Here's how the part is built. I have some questions about the finished solid (model axes, mm). Face numbers are marked on the shaded views. Coordinates: 2 decimals unless noted, no trailing zeros. Loops run counter-clockwise (first coordinate to the right, second up) from the corner with the lowest first, then second, coordinate; pieces in that order, holes last.
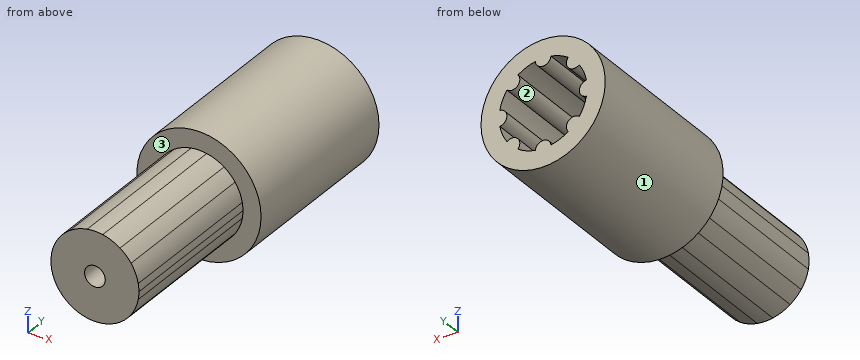
```python
from build123d import *

# Parameters (mm, degrees)
F0_R          = 6
F1_DEPTH      = 17
F0_R_2        = 2.5
F0_R_3        = 1
F2_DEPTH      = 15
F2_DEPTH_BACK = 3


with BuildPart() as f1:
    # F0 (on Front) → F1 (new body)
    with BuildSketch(Plane.XZ):
        Circle(F0_R)
        with BuildLine():
            ThreePointArc((4.183153, 0.75082), (4.233255, 0.376895), (4.25, 0))
            ThreePointArc((4.25, 0), (4.233255, -0.376895), (4.183153, -0.75082))
            ThreePointArc((4.183153, -0.75082), (3.926488, -1.626405), (3.488846, -2.427026))
            ThreePointArc((3.488846, -2.427026), (3.005204, -3.005204), (2.427026, -3.488846))
            ThreePointArc((2.427026, -3.488846), (1.626405, -3.926488), (0.75082, -4.183153))
            ThreePointArc((0.75082, -4.183153), (0, -4.25), (-0.75082, -4.183153))
            ThreePointArc((-0.75082, -4.183153), (-1.626405, -3.926488), (-2.427026, -3.488846))
            ThreePointArc((-2.427026, -3.488846), (-3.005204, -3.005204), (-3.488846, -2.427026))
            ThreePointArc((-3.488846, -2.427026), (-3.926488, -1.626405), (-4.183153, -0.75082))
            ThreePointArc((-4.183153, -0.75082), (-4.25, 0), (-4.183153, 0.75082))
            ThreePointArc((-4.183153, 0.75082), (-3.926488, 1.626405), (-3.488846, 2.427026))
            ThreePointArc((-3.488846, 2.427026), (-3.005204, 3.005204), (-2.427026, 3.488846))
            ThreePointArc((-2.427026, 3.488846), (-1.626405, 3.926488), (-0.75082, 4.183153))
            ThreePointArc((-0.75082, 4.183153), (0, 4.25), (0.75082, 4.183153))
            ThreePointArc((0.75082, 4.183153), (1.626405, 3.926488), (2.427026, 3.488846))
            ThreePointArc((2.427026, 3.488846), (3.005204, 3.005204), (3.488846, 2.427026))
            ThreePointArc((3.488846, 2.427026), (3.926488, 1.626405), (4.183153, 0.75082))
        make_face(mode=Mode.SUBTRACT)
        with BuildLine():
            ThreePointArc((4.183153, -0.75082), (4.233255, -0.376895), (4.25, 0))
            ThreePointArc((4.25, 0), (4.233255, 0.376895), (4.183153, 0.75082))
            ThreePointArc((4.183153, 0.75082), (3.496211, 0), (4.183153, -0.75082))
        make_face()
        with BuildLine():
            ThreePointArc((2.427026, 3.488846), (2.472194, 2.472194), (3.488846, 2.427026))
            ThreePointArc((3.488846, 2.427026), (3.005204, 3.005204), (2.427026, 3.488846))
        make_face()
        with BuildLine():
            ThreePointArc((-0.75082, 4.183153), (0, 3.496211), (0.75082, 4.183153))
            ThreePointArc((0.75082, 4.183153), (0, 4.25), (-0.75082, 4.183153))
        make_face()
        with BuildLine():
            ThreePointArc((-3.488846, 2.427026), (-2.472194, 2.472194), (-2.427026, 3.488846))
            ThreePointArc((-2.427026, 3.488846), (-3.005204, 3.005204), (-3.488846, 2.427026))
        make_face()
        with BuildLine():
            ThreePointArc((-4.183153, -0.75082), (-3.496211, 0), (-4.183153, 0.75082))
            ThreePointArc((-4.183153, 0.75082), (-4.25, 0), (-4.183153, -0.75082))
        make_face()
        with BuildLine():
            ThreePointArc((-3.488846, -2.427026), (-3.005204, -3.005204), (-2.427026, -3.488846))
            ThreePointArc((-2.427026, -3.488846), (-2.472194, -2.472194), (-3.488846, -2.427026))
        make_face()
        with BuildLine():
            ThreePointArc((-0.75082, -4.183153), (0, -4.25), (0.75082, -4.183153))
            ThreePointArc((0.75082, -4.183153), (0, -3.496211), (-0.75082, -4.183153))
        make_face()
        with BuildLine():
            ThreePointArc((2.427026, -3.488846), (3.005204, -3.005204), (3.488846, -2.427026))
            ThreePointArc((3.488846, -2.427026), (2.472194, -2.472194), (2.427026, -3.488846))
        make_face()
    extrude(amount=-F1_DEPTH)

    # F0 (on Front) → F2 (join, two sides)
    with BuildSketch(Plane.XZ) as f2_sk:
        with BuildLine():
            ThreePointArc((4.183153, -0.75082), (3.496211, 0), (4.183153, 0.75082))
            ThreePointArc((4.183153, 0.75082), (3.926488, 1.626405), (3.488846, 2.427026))
            ThreePointArc((3.488846, 2.427026), (2.472194, 2.472194), (2.427026, 3.488846))
            ThreePointArc((2.427026, 3.488846), (1.626405, 3.926488), (0.75082, 4.183153))
            ThreePointArc((0.75082, 4.183153), (0, 3.496211), (-0.75082, 4.183153))
            ThreePointArc((-0.75082, 4.183153), (-1.626405, 3.926488), (-2.427026, 3.488846))
            ThreePointArc((-2.427026, 3.488846), (-2.472194, 2.472194), (-3.488846, 2.427026))
            ThreePointArc((-3.488846, 2.427026), (-3.926488, 1.626405), (-4.183153, 0.75082))
            ThreePointArc((-4.183153, 0.75082), (-3.496211, 0), (-4.183153, -0.75082))
            ThreePointArc((-4.183153, -0.75082), (-3.926488, -1.626405), (-3.488846, -2.427026))
            ThreePointArc((-3.488846, -2.427026), (-2.472194, -2.472194), (-2.427026, -3.488846))
            ThreePointArc((-2.427026, -3.488846), (-1.626405, -3.926488), (-0.75082, -4.183153))
            ThreePointArc((-0.75082, -4.183153), (0, -3.496211), (0.75082, -4.183153))
            ThreePointArc((0.75082, -4.183153), (1.626405, -3.926488), (2.427026, -3.488846))
            ThreePointArc((2.427026, -3.488846), (2.472194, -2.472194), (3.488846, -2.427026))
            ThreePointArc((3.488846, -2.427026), (3.926488, -1.626405), (4.183153, -0.75082))
        make_face()
        Circle(F0_R_2, mode=Mode.SUBTRACT)
        Circle(F0_R_2)
        Circle(F0_R_3, mode=Mode.SUBTRACT)
        with BuildLine():
            ThreePointArc((-3.488846, 2.427026), (-2.472194, 2.472194), (-2.427026, 3.488846))
            ThreePointArc((-2.427026, 3.488846), (-3.005204, 3.005204), (-3.488846, 2.427026))
        make_face()
        with BuildLine():
            ThreePointArc((-4.183153, -0.75082), (-3.496211, 0), (-4.183153, 0.75082))
            ThreePointArc((-4.183153, 0.75082), (-4.25, 0), (-4.183153, -0.75082))
        make_face()
        with BuildLine():
            ThreePointArc((-3.488846, -2.427026), (-3.005204, -3.005204), (-2.427026, -3.488846))
            ThreePointArc((-2.427026, -3.488846), (-2.472194, -2.472194), (-3.488846, -2.427026))
        make_face()
        with BuildLine():
            ThreePointArc((-0.75082, -4.183153), (0, -4.25), (0.75082, -4.183153))
            ThreePointArc((0.75082, -4.183153), (0, -3.496211), (-0.75082, -4.183153))
        make_face()
        with BuildLine():
            ThreePointArc((2.427026, -3.488846), (3.005204, -3.005204), (3.488846, -2.427026))
            ThreePointArc((3.488846, -2.427026), (2.472194, -2.472194), (2.427026, -3.488846))
        make_face()
        with BuildLine():
            ThreePointArc((2.427026, 3.488846), (2.472194, 2.472194), (3.488846, 2.427026))
            ThreePointArc((3.488846, 2.427026), (3.005204, 3.005204), (2.427026, 3.488846))
        make_face()
        with BuildLine():
            ThreePointArc((-0.75082, 4.183153), (0, 3.496211), (0.75082, 4.183153))
            ThreePointArc((0.75082, 4.183153), (0, 4.25), (-0.75082, 4.183153))
        make_face()
        with BuildLine():
            ThreePointArc((4.183153, -0.75082), (4.233255, -0.376895), (4.25, 0))
            ThreePointArc((4.25, 0), (4.233255, 0.376895), (4.183153, 0.75082))
            ThreePointArc((4.183153, 0.75082), (3.496211, 0), (4.183153, -0.75082))
        make_face()
    extrude(amount=F2_DEPTH)
    extrude(f2_sk.sketch, amount=-F2_DEPTH_BACK)


solid = f1.part
```
1. I need wall thicknesses on line 1 along Z through (x, y) = (0, 1.85); line 2 along Y through (x, z) = (3, 0.5); line 3 along Z through (x, y) = (-1, 9). Which ranges of each line are inside material? Lowest first, please.
2. I want a section at B-B (x = 0). Please give me the cut outline in (y, z).
3. We'd pull the mould along Z, two halves only. Please class the marked faces 1, 2 and 3: +Z half, -Z half, draft (parallel to the pull), parting line (faces both ways), or undercut.
4. For pin 1 (3 mm diameter, centred on x = -0.5, z = -2, fed in from +Y); pin 2 (3 mm diameter, centred on x = -1, y = -7.5, fed in from -Z), each with a flat end and sliding along its axis, tell me the tip position at first contact or that it passes through.
5. I want a section at A-A (y = 5.5). Please give me the cut outline in (x, z).
6. I want a section at C-C (z = -2.75). Please give me the cut outline in (x, y), then the cut area to 3 significant figures.
7. I want a section at D-D (y = -2). Please give me the cut outline in (x, z), then the cut area to 3 significant figures.
Response values:
1. line 1: z = -6 to -1, 1 to 6
1. line 2: y = -15 to 3
1. line 3: z = -5.92 to -4.13, 4.13 to 5.92
2. outline: (-15, -4.25) - (0, -4.25) - (0, -6) - (17, -6) - (17, -3.5) - (3, -3.5) - (3, -1) - (-15, -1) - close; (-15, 1) - (3, 1) - (3, 3.5) - (17, 3.5) - (17, 6) - (0, 6) - (0, 4.25) - (-15, 4.25) - close
3. face 1: parting line
3. face 2: undercut
3. face 3: draft
4. pin 1: stops at y = 3
4. pin 2: stops at z = -4.25
5. outline: circle Ø12 at (0, 0); hole (-4.18, -0.75) arc R4.25 ccw to (-3.49, -2.43) arc R0.75 cw to (-2.43, -3.49) arc R4.25 ccw to (-0.75, -4.18) arc R0.75 cw to (0.75, -4.18) arc R4.25 ccw to (2.43, -3.49) arc R0.75 cw to (3.49, -2.43) arc R4.25 ccw to (4.18, -0.75) arc R0.75 cw to (4.18, 0.75) arc R4.25 ccw to (3.49, 2.43) arc R0.75 cw to (2.43, 3.49) arc R4.25 ccw to (0.75, 4.18) arc R0.75 cw to (-0.75, 4.18) arc R4.25 ccw to (-2.43, 3.49) arc R0.75 cw to (-3.49, 2.43) arc R4.25 ccw to (-4.18, 0.75) arc R0.75 cw to start
6. outline: (-5.33, 0) - (-3.24, 0) - (-3.24, -15) - (3.24, -15) - (3.24, 0) - (5.33, 0) - (5.33, 17) - (2.3, 17) - (2.3, 3) - (-2.3, 3) - (-2.3, 17) - (-5.33, 17) - close
6. area: 214 mm2
7. outline: (-4.18, -0.75) arc R4.25 ccw to (-3.49, -2.43) arc R4.25 ccw to (-2.43, -3.49) arc R4.25 ccw to (-0.75, -4.18) arc R4.25 ccw to (0.75, -4.18) arc R4.25 ccw to (2.43, -3.49) arc R4.25 ccw to (3.49, -2.43) arc R4.25 ccw to (4.18, -0.75) arc R4.25 ccw to (4.25, 0) arc R4.25 ccw to (4.18, 0.75) arc R4.25 ccw to (3.49, 2.43) arc R4.25 ccw to (2.43, 3.49) arc R4.25 ccw to (0.75, 4.18) arc R4.25 ccw to (-0.75, 4.18) arc R4.25 ccw to (-2.43, 3.49) arc R4.25 ccw to (-3.49, 2.43) arc R4.25 ccw to (-4.18, 0.75) arc R4.25 ccw to start; hole circle Ø2 at (0, 0)
7. area: 53.6 mm2
